Autodesk Inventor part; units mm, degrees
ref_plane "YZ Plane" through (0, 0, 0) normal (1, 0, 0) x (0, 1, 0)
ref_plane "XZ Plane" through (0, 0, 0) normal (0, 1, 0) x (-1, 0, 0)
ref_plane "XY Plane" through (0, 0, 0) normal (0, 0, 1) x (1, 0, 0)
sketch "스케치2" plane through (0, 0, 0) normal (0, 1, 0) x (-1, 0, 0)
  line L0 (0, 60) -> (51.9615, 30)
  line L1 (51.9615, 30) -> (51.9615, -30)
  line L2 (51.9615, -30) -> (0, -60)
  line L3 (0, -60) -> (-51.9615, -30)
  line L4 (-51.9615, -30) -> (-51.9615, 30)
  line L5 (-51.9615, 30) -> (0, 60)
  line L6 (0, 65.7735) -> (56.9615, 32.8868)
  line L7 (56.9615, 32.8868) -> (56.9615, -32.8868)
  line L8 (56.9615, -32.8868) -> (0, -65.7735)
  line L9 (0, -65.7735) -> (-56.9615, -32.8868)
  line L10 (-56.9615, -32.8868) -> (-56.9615, 32.8868)
  line L11 (-56.9615, 32.8868) -> (0, 65.7735)
  circle A0 centre (-54.4615, 0) radius 2.5 construction
  circle A1 centre (-54.4615, 0) radius 2.6
  circle A2 centre (-27.2308, -47.1651) radius 2.5 construction
  circle A3 centre (-27.2308, -47.1651) radius 2.6
  circle A4 centre (27.2308, -47.1651) radius 2.5 construction
  circle A5 centre (27.2308, -47.1651) radius 2.6
  circle A6 centre (54.4615, 0) radius 2.5 construction
  circle A7 centre (54.4615, 0) radius 2.6
  circle A8 centre (27.2308, 47.1651) radius 2.5 construction
  circle A9 centre (27.2308, 47.1651) radius 2.6
  circle A10 centre (-27.2308, 47.1651) radius 2.5 construction
  circle A11 centre (-27.2308, 47.1651) radius 2.6
  point P0 (0, 0)
  point P1 (0, 0)
  point P2 (-56.9615, -0.7141)
  point P3 (-29.0992, -48.9731)
  point P4 (-27.8623, -49.6872)
  point P5 (27.8623, -49.6872)
  point P6 (29.0992, -48.9731)
  point P7 (56.9615, -0.7141)
  point P8 (56.9615, 0.7141)
  point P9 (29.0992, 48.9731)
  point P10 (27.8623, 49.6872)
  point P11 (-27.8623, 49.6872)
  point P12 (-29.0992, 48.9731)
  point P13 (-56.9615, 0.7141)
  point P14 (25.3623, -45.3571)
  point P15 (26.5992, -44.6429)
  dimension "d0" = 60
  dimension "d1" = 5
  dimension "d2" = 5
  dimension "d3" = 5.2
  dimension "d6" = 360
extrude "돌출1" add sketch "스케치2" along normal blind 5 contours L5 A11 L11 L6 A9 L0 | L0 A9 L1 A7 L2 A5 L3 A3 L4 A1 L5 A11 | A9 L6 L7 A7 L1 L0 | L5 L4 A1 L10 L11 A11 | A7 L7 L1 | L1 A7 | A1 L4 | L4 A1 L10 | A7 L7 L8 A5 L2 L1 | L4 L3 A3 L9 L10 A1 | L2 A5 | A5 L8 L9 A3 L3 L2
fillet "모깎기1" radius 1 8 edges at (-29.0992, 2.5, 48.9731) (-27.8623, 2.5, 49.6872) (27.8623, 2.5, 49.6872) (29.0992, 2.5, 48.9731) (27.8623, 2.5, -49.6872) (29.0992, 2.5, -48.9731) (-29.0992, 2.5, -48.9731) (-27.8623, 2.5, -49.6872)
sketch "스케치3" plane through (0, 5, 0) normal (0, 1, 0) x (1, 0, 0)
  circle A0 centre (0, 0) radius 2.5
  line L0 (0, 10) -> (8.6603, 5)
  line L1 (8.6603, 5) -> (8.6603, -5)
  line L2 (8.6603, -5) -> (0, -10)
  line L3 (0, -10) -> (-8.6603, -5)
  line L4 (-8.6603, -5) -> (-8.6603, 5)
  line L5 (-8.6603, 5) -> (0, 10)
  line L6 (0, 20) -> (17.3205, 10)
  line L7 (17.3205, 10) -> (17.3205, -10)
  line L8 (17.3205, -10) -> (0, -20)
  line L9 (0, -20) -> (-17.3205, -10)
  line L10 (-17.3205, -10) -> (-17.3205, 10)
  line L11 (-17.3205, 10) -> (0, 20)
  line L12 (0, 30) -> (25.9808, 15)
  line L13 (25.9808, 15) -> (25.9808, -15)
  line L14 (25.9808, -15) -> (0, -30)
  line L15 (0, -30) -> (-25.9808, -15)
  line L16 (-25.9808, -15) -> (-25.9808, 15)
  line L17 (-25.9808, 15) -> (0, 30)
  circle A1 centre (0, 10) radius 2.5
  circle A2 centre (0, 20) radius 2.5
  circle A3 centre (0, 30) radius 2.5
  circle A4 centre (-25.9808, 15) radius 2.5
  circle A5 centre (-17.3205, 10) radius 2.5
  circle A6 centre (-8.6603, 5) radius 2.5
  circle A7 centre (-25.9808, -15) radius 2.5
  circle A8 centre (-17.3205, -10) radius 2.5
  circle A9 centre (-8.6603, -5) radius 2.5
  circle A10 centre (0, -30) radius 2.5
  circle A11 centre (0, -20) radius 2.5
  circle A12 centre (0, -10) radius 2.5
  circle A13 centre (25.9808, -15) radius 2.5
  circle A14 centre (17.3205, -10) radius 2.5
  circle A15 centre (8.6603, -5) radius 2.5
  circle A16 centre (25.9808, 15) radius 2.5
  circle A17 centre (17.3205, 10) radius 2.5
  circle A18 centre (8.6603, 5) radius 2.5
  dimension "d11" = 5
  dimension "d12" = 10
  dimension "d13" = 20
  dimension "d14" = 30
  dimension "d17" = 360
extrude "돌출2" cut sketch "스케치3" against normal through all contours A0 | L5 A1 L0 | L0 A1 L5 | A18 L1 L0 | L0 L1 A18 | A6 L4 L5 | L5 L4 A6 | A15 L2 L1 | L1 L2 A15 | A9 L3 L4 | L4 L3 A9 | A12 L3 L2 | L2 L3 A12 | L11 A2 L6 | L6 A2 L11 | A17 L7 L6 | L6 L7 A17 | A5 L10 L11 | L11 L10 A5 | A14 L8 L7 | L7 L8 A14 | A8 L9 L10 | L10 L9 A8 | A11 L9 L8 | L8 L9 A11 | L17 A3 L12 | L12 A3 L17 | A16 L13 L12 | L12 L13 A16 | A4 L16 L17 | L17 L16 A4 | A13 L14 L13 | L13 L14 A13 | A7 L15 L16 | L16 L15 A7 | A10 L15 L14 | L14 L15 A10
properties part number "top"
Model file for the job. Use its own axes, mm. A direction names the side the tool comes from. Round coordinates to 2 decimals unless told otherwise and drop trailing zeros. Order: outer loops, then holes, each group sorted by start corner. A loop starts at its lowest first (then second) coordinate and runs counter-clockwise, first axis right, second up. Notation, with made-up numbers: M -40,-27 L 6,-27 A28 ccw 6,3 Z; hole C 24,53.5 d11. An arc over 180 degrees is marked long. Use CSV: the item, a comma, the result in double quotes.
Item 1: Saw through at B-B (z = 30). List the corners of the cut face in (x, y).
Worked answers:
outline,"M -56.96,0 L -2.5,0 L -2.5,5 L -56.96,5 Z; M 2.5,0 L 56.96,0 L 56.96,5 L 2.5,5 Z"
Item 2: Pull direction Z, two halves, no side cores. Call faces 3 (the face through (-56.962, 2, 0)), 4 (the face through (-25.99, 2.46, 44.88)), 5 (the face through (-0.33, 2.54, 27.52)), 6 (the face through (13, 2.46, 58.27)): released by +Z, released by -Z, zero draft, split by the parting line, or undercut.
Worked answers:
face 3,"zero draft"
face 4,"undercut"
face 5,"undercut"
face 6,"released by +Z"
Item 3: Which spindle directions (+Z, -Z, +X, -X, +Y, -Y) get a long thin tool onto all of the face, cutting with end or side? Do faces 1 (the face through (-24.645, 2.465, -47.436)), 2 (the face through (56.962, 2, 0)). Say none if no direction does.
Worked answers:
face 1,"+Y, -Y"
face 2,"+Z, -Z, +X, +Y, -Y"
Item 4: Saw through at C-C (y = 1.25). State how many separate pieces and enclosed holes the cut face has, plus the area to 3 significant figures.
Worked answers:
separate pieces,"1"
enclosed holes,"19"
area,"10,800 mm²"
Item 5: Probe probe 1 along X at (y, z) = (1.9, 10); probe 2 along X at (y, z) = (1.45, 5); probe 3 along Z at (x, y) = (-16, 4.3). List the from-to ranges inside material, lowest first.
Worked answers:
probe 1,"-56.96 to -19.82, -14.82 to -2.5, 2.5 to 14.82, 19.82 to 56.96"
probe 2,"-56.96 to -11.16, -6.16 to 6.16, 11.16 to 56.96"
probe 3,"-56.54 to -12.12, -7.88 to 7.88, 12.12 to 56.54"
Item 6: Saw through at A-A (z = -15). List the corners of the cut face in (x, y), plus the area to 3 significant figures.
Worked answers:
outline,"M -56.96,0 L -28.48,0 L -28.48,5 L -56.96,5 Z; M -23.48,0 L 23.48,0 L 23.48,5 L -23.48,5 Z; M 28.48,0 L 56.96,0 L 56.96,5 L 28.48,5 Z"
area,"520 mm²"
Item 7: Saw through at D-D (z = -40). List the corners of the cut face in (x, y), plus the area to 3 significant figures.
Worked answers:
outline,"M -44.64,0 L 44.64,0 L 44.64,5 L -44.64,5 Z"
area,"446 mm²"
